For this review, use the dimensioned drawing (mm, ordinates from the lowest corner) and the shaded views. Round coordinates to 2 decimals unless told otherwise and drop trailing zeros. Write each loop counter-clockwise with the first axis right and the second up, starting at its lowest first coordinate (ties: lowest second). Pieces come first, ordered by that corner, then holes.
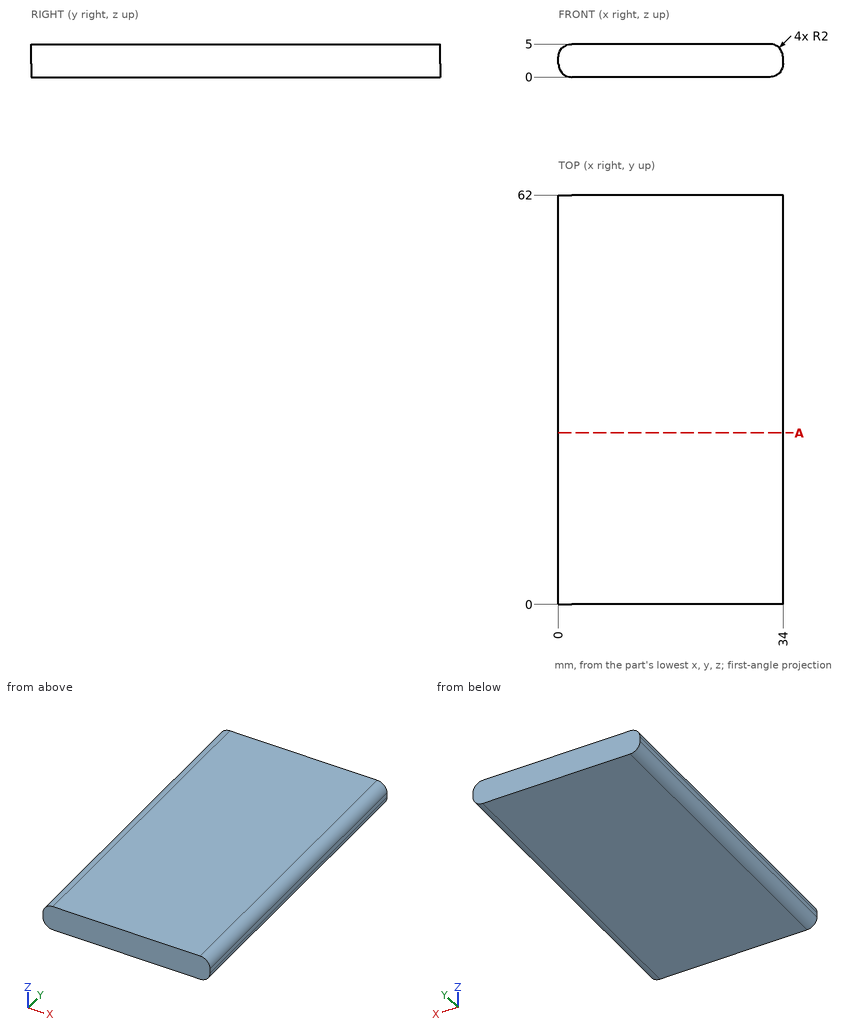
(1) For line 1 along X through (y, z) = (45, 1.85); line 2 along X through (y, z) = (29, 4.8), list the stretches that pass through material, from the lowest coordinate up.
Geometry check:
line 1: x = 0.01 to 33.99
line 2: x = 1.13 to 32.87
(2) For pin 1 Ø1.5 at (y, z) = (55.5, 0.5) entering from -X, flat-tipped, find the tip position at first contact; note if it passes through.
Geometry check:
pin 1: stops at x = 0.15
(3) We need section A-A, the plane y = 26. Give the boundary of the cut face in (x, z), and give its area (3 significant figures).
Geometry check:
outline: (0, 2) arc R2 ccw to (2, 0) - (32, 0) arc R2 ccw to (34, 2) - (34, 3) arc R2 ccw to (32, 5) - (2, 5) arc R2 ccw to (0, 3) - close
area: 167 mm2
